Source: CAD feature listing. Evaluate the final solid. Frame: model axes, mm. A direction names the side the tool comes from. Round coordinates to 2 decimals unless told otherwise and drop trailing zeros. Loops run counter-clockwise (first coordinate to the right, second up) from the corner with the lowest first, then second, coordinate; pieces in that order, holes last. Notation, with made-up numbers: (-26, 7.25) -> (7, 7.25) arc R15 ccw to (7, 14.25) -> close; hole circle Ø3 at (51.5, 58). An arc over 180 degrees is marked (long way). Put each result on its own line as item: value. Start each with the question number.
1. Cut plane D-D (z = -11.25). Return the cut outline in (x, y) (3 decimals), then the cut area to 4 significant figures.
2. Material intervals for L1, parallel to Y at x = 1.15, z = -7; L2, parallel to Z at x = 9, y = 28 (3 decimals); L3, parallel to X at y = 11, z = -1.25 (3 decimals), sorted ascending.
3. Draft query along Z for faces 3 (the cylindrical face through (24.004, 6.816, -20.39)), 4 (the flat face through (20.4, 18.2, -18.825)), 5 (the cylindrical face through (1.61, 21.85, -9.77)), 6 (the cylindrical face through (1.61, 5.85, -9.77)). Return one class per face: pulls with the +Z half, pulls with the -Z half, needs draft (parallel to the pull), parting line crosses it, or undercut.
4. Set-up query: faces 1 (the flat face through (0, 15, -8)), 2 (the flat face through (3.175, 15, -7)). Return all of +Z, -Z, +X, -X, +Y, -Y with unobstructed straight access to the full face (end or side cutting, diameter ignored); none if empty.
5. Contact query for flat-ended pins moving along their axis: pin 1 (11 mm diameter, centred on y = 11, z = -9.5, fed in from +X) (3 decimals); pin 2 (5.5 mm diameter, centred on y = 23, z = -7, fed in from +X); pin 3 (2 mm diameter, centred on y = 19, z = -18.5, fed in from -X); pin 4 (7 mm diameter, centred on y = 7, z = -7, fed in from +X) (3 decimals). Output: stop coordinate, or through.
6. Cut plane C-C (x = 14). Return the cut outline in (y, z) (3 decimals), then the cut area to 3 significant figures.
7. Cut plane A-A (y = 15). Return the cut outline in (x, z) (3 decimals), then the cut area to 3 significant figures.
8. Cut plane B-B (z = -5.75). Return the cut outline in (x, y) (3 decimals).
```python
from build123d import *

# Parameters (mm, degrees)
SKETCH1_W           = 22
SKETCH1_H           = 30
BOSS_EXTRUDE1_DEPTH = 3.175
SKETCH2_W           = 25
SKETCH2_H           = 30
BOSS_EXTRUDE2_DEPTH = 3.175
SKETCH3_R           = 6
CUT_EXTRUDE1_DEPTH  = 45.821869662
CUT_EXTRUDE4_REACH  = 46.822
FILLET1_R           = 5
SKETCH4_R           = 3
CUT_EXTRUDE2_DEPTH  = 44.131550227


with BuildPart() as part:
    # Sketch1 → Boss-Extrude1 (new body)
    with BuildSketch(Plane(origin=(0, 0, 0), x_dir=(0, 0, -1), z_dir=(1, 0, 0))):
        with Locations((11, 15)):
            Rectangle(SKETCH1_W, SKETCH1_H)
    extrude(amount=BOSS_EXTRUDE1_DEPTH)

    # Sketch2 → Boss-Extrude2 (add)
    with BuildSketch(Plane(origin=(0, 0, -22), x_dir=(-1, 0, 0), z_dir=(0, 0, -1))):
        with Locations((-12.5, 15)):
            Rectangle(SKETCH2_W, SKETCH2_H)
    extrude(amount=-BOSS_EXTRUDE2_DEPTH)

    # Sketch3 → Cut-Extrude1 (cut, through all)
    with BuildSketch(Plane(origin=(0, 0, -22), x_dir=(-1, 0, 0), z_dir=(0, 0, -1))):
        with Locations((-15, 15)):
            Circle(SKETCH3_R)
    extrude(amount=-CUT_EXTRUDE1_DEPTH, mode=Mode.SUBTRACT)

    # Sketch5 → Cut-Extrude4 (cut, up to next)
    with BuildSketch(Plane(origin=(0, 0, -22), x_dir=(-1, 0, 0), z_dir=(0, 0, -1)), mode=Mode.PRIVATE) as cut_extrude4_sk1:
        Polygon((-3.175, 30), (-25, 24), (-25, 30), align=None)
    cut_extrude4_tool1 = extrude(cut_extrude4_sk1.sketch, amount=-CUT_EXTRUDE4_REACH, mode=Mode.PRIVATE) & part.part
    # Sketch5 → Cut-Extrude4 (cut, up to next)
    with BuildSketch(Plane(origin=(0, 0, -22), x_dir=(-1, 0, 0), z_dir=(0, 0, -1)), mode=Mode.PRIVATE) as cut_extrude4_sk2:
        Polygon((-25, 0), (-3.175, 0), (-25, 6), align=None)
    cut_extrude4_tool2 = extrude(cut_extrude4_sk2.sketch, amount=-CUT_EXTRUDE4_REACH, mode=Mode.PRIVATE) & part.part
    add(cut_extrude4_tool1.solids().sort_by_distance((17.725, 28, -22))[0], mode=Mode.SUBTRACT)
    add(cut_extrude4_tool2.solids().sort_by_distance((17.725, 2, -22))[0], mode=Mode.SUBTRACT)

    # Fillet1
    fillet1_edges = [part.edges().sort_by_distance(p)[0] for p in [
        (1.5875, 30, 0),
        (1.5875, 0, 0),
        (0, 15, -22),
        (3.175, 15, -18.825),
        (25, 6, -20.4125),
        (25, 24, -20.4125),
    ]]
    fillet(fillet1_edges, radius=FILLET1_R)

    # Sketch4 → Cut-Extrude2 (cut, through all)
    with BuildSketch(Plane(origin=(3.175, 0, 0), x_dir=(0, 0, -1), z_dir=(1, 0, 0))):
        with Locations((7, 23)):
            Circle(SKETCH4_R)
        with Locations((7, 7)):
            Circle(SKETCH4_R)
    extrude(amount=-CUT_EXTRUDE2_DEPTH, mode=Mode.SUBTRACT)


solid = part.part
```
Solution:
1. outline: (0, 0) -> (3.175, 0) -> (3.175, 30) -> (0, 30) -> close
1. area: 95.25 mm^2
2. L1: y = 0 to 4, 10 to 20, 26 to 30
2. L2: z = -22 to -18.825
2. L3: x = 0 to 3.175
3. face 3: needs draft
3. face 4: pulls with the +Z half
3. face 5: undercut
3. face 6: undercut
4. face 1: +Z, -Z, -X, +Y, -Y
4. face 2: +Z, +X, +Y, -Y
5. pin 1: stops at x = 3.315
5. pin 2: passes through
5. pin 3: stops at x = 0.03
5. pin 4: stops at x = 3.175
6. outline: (2.976, -22) -> (9.084, -22) -> (9.084, -18.825) -> (2.976, -18.825) -> close; (20.916, -22) -> (27.024, -22) -> (27.024, -18.825) -> (20.916, -18.825) -> close
6. area: 38.8 mm^2
7. outline: (0, -17) arc R5 ccw to (5, -22) -> (9, -22) -> (9, -18.825) -> (8.175, -18.825) arc R5 cw to (3.175, -13.825) -> (3.175, 0) -> (0, 0) -> close; (21, -22) -> (25, -22) -> (25, -18.825) -> (21, -18.825) -> close
7. area: 101 mm^2
8. outline: (0, 0) -> (3.175, 0) -> (3.175, 4.273) -> (0, 4.273) -> close; (0, 9.727) -> (3.175, 9.727) -> (3.175, 20.273) -> (0, 20.273) -> close; (0, 25.727) -> (3.175, 25.727) -> (3.175, 30) -> (0, 30) -> close
